Geometry check sheet. Reference: the model listing, model coordinates, mm. A direction names the side the tool comes from. Coordinates: 2 decimals unless noted, no trailing zeros. Loops run counter-clockwise (first coordinate to the right, second up) from the corner with the lowest first, then second, coordinate; pieces in that order, holes last.
from build123d import *

# Parameters (mm, degrees)
EXTRUDE_1_DEPTH            = 1.27
EXTRUDE_2_DEPTH            = 0.01
EXTRUDE_2_DEPTH_BACK       = 10.17
SKETCH_4_R                 = 0.51
SKETCH_4_R_2               = 0.5
CUT_EXTRUDE_1_DEPTH        = 0.1
EXTRUDE_3_DEPTH            = 0.485
PATTERN_LINEAR_1_COUNT     = 3
PATTERN_LINEAR_1_PITCH     = 1.7
PATTERN_LINEAR_1_COL_COUNT = 3
PATTERN_LINEAR_1_COL_PITCH = 1.7


with BuildPart() as part:
    # Эскиз2 → Бобышка-Вытянуть1 (new body)
    with BuildSketch(Plane(origin=(0, 0, 0), x_dir=(1, 0, 0), z_dir=(0, 1, 0))):
        Polygon((3.43, 6.35), (5.08, 6.059060482), (5.08, 5.08), (2.9, 5.08), (2.9, 0), (-2.9, 0), (-2.9, 5.08), (-5.08, 5.08), (-5.08, 6.059060482), (-3.43, 6.35), align=None)
    extrude(amount=EXTRUDE_1_DEPTH)

    # Эскиз3 → Бобышка-Вытянуть2 (add, two sides: drawn at the far end of the back side and taken through both)
    with BuildSketch(Plane.ZY.offset(5.08).offset(-EXTRUDE_2_DEPTH_BACK)):
        Polygon((-5.08, 0.01), (-5.08, 1.27), (-4.673583103, 4.58), (3.357405475, 4.58), (3.56, 2.93), (3.56, 2.55), (3.248127215, 0.01), align=None)
    extrude(amount=EXTRUDE_2_DEPTH + EXTRUDE_2_DEPTH_BACK)

    # Эскиз4 → Вырез-Вытянуть1 (cut)
    with BuildSketch(Plane(origin=(0, 4.58, 0), x_dir=(1, 0, 0), z_dir=(0, 1, 0))):
        with Locations(Location((-3.59, -1.857405475, 0), (0, 0, 270))):
            Circle(SKETCH_4_R)
        with Locations(Location((-3.59, -1.857405475, 0), (0, 0, 270))):
            Circle(SKETCH_4_R_2, mode=Mode.SUBTRACT)
    extrude(amount=-CUT_EXTRUDE_1_DEPTH, mode=Mode.SUBTRACT)

    # Эскиз5 → Бобышка-Вытянуть3 (add, symmetric)
    with BuildSketch(Plane(origin=(0, 0, 0), x_dir=(0, 0, -1), z_dir=(1, 0, 0))):
        with BuildLine():
            Line((-3.56, 2.93), (-3.56, 2.55))
            Line((-3.56, 2.55), (-5.067677126, 2.55))
            ThreePointArc((-5.067677126, 2.55), (-5.576216387, 2.354790067), (-5.823513767, 1.869441632))
            Line((-5.823513767, 1.869441632), (-5.948470433, 0.680558368))
            ThreePointArc((-5.948470433, 0.680558368), (-6.195767813, 0.195209933), (-6.704307074, 0))
            Line((-6.704307074, 0), (-8, 0))
            Line((-8, 0), (-8, 0.38))
            Line((-8, 0.38), (-6.704307074, 0.38))
            ThreePointArc((-6.704307074, 0.38), (-6.450037443, 0.477604966), (-6.326388753, 0.720279184))
            Line((-6.326388753, 0.720279184), (-6.201432087, 1.909162448))
            ThreePointArc((-6.201432087, 1.909162448), (-5.830486018, 2.637185101), (-5.067677126, 2.93))
            Line((-5.067677126, 2.93), (-3.56, 2.93))
        make_face()
    extrude_3 = extrude(amount=EXTRUDE_3_DEPTH, both=True)

    # Линейный массив1: Бобышка-Вытянуть3 ×3
    with Locations(*[(-i * PATTERN_LINEAR_1_PITCH, 0, 0) for i in range(1, PATTERN_LINEAR_1_COUNT)]):
        add(extrude_3)

    # Линейный массив1 col: Бобышка-Вытянуть3 ×3
    with Locations(*[(i * PATTERN_LINEAR_1_COL_PITCH, 0, 0) for i in range(1, PATTERN_LINEAR_1_COL_COUNT)]):
        add(extrude_3)


solid = part.part
(1) Scan lines: L1, parallel to Y at x = 4.75, z = 3; L2, parallel to Y at x = 1.25, z = 3.75; L3, parallel to Z at x = -2, y = 0.75. Record each from-to range of solid material in increasing order.
Findings:
L1: y = 0.01 to 4.58
L2: y = 2.55 to 2.93
L3: z = -6.35 to 3.34, 5.94 to 6.32
(2) Gauge pin test, flat ends, axial feed: pin 1 Ø1.1 at (x, z) = (-3.5, 4.5) entering from +Y; pin 2 Ø1.5 at (y, z) = (1, 5.5) entering from -X (3 decimals); pin 3 Ø0.5 at (x, z) = (-2, 4.5) entering from -Y. Record the tip position at first contact, or that the pin passes through.
Findings:
pin 1: stops at y = 2.93
pin 2: stops at x = -3.885
pin 3: stops at y = 2.55
(3) Access from +Z, -Z, +X, -X, +Y, -Y to the whole of each face (thin tool, end or side, straight path). Record for faces 4 (the flat face through (-3.4, 0.38, 7.4)), 5 (the flat face through (2, 0, 7)), 6 (the flat face through (2, 2.55, 4)), 7 (the flat face through (3.885, 2, 6)), 8 (the flat face through (-3.885, 2, 6)).
Findings:
face 4: +Z, +X, -X, +Y
face 5: +Z, -Z, +X, -X, -Y
face 6: +X, -X, -Y
face 7: +Z, +X, +Y, -Y
face 8: +Z, -X, +Y, -Y
(4) Sectioned sample at A-A on y = 2.1. Record the cut outline in (x, z) (3 decimals).
Findings:
outline: (-5.09, -4.978) - (5.09, -4.978) - (5.09, 3.505) - (-5.09, 3.505) - close; (-3.885, 5.762) - (-2.915, 5.762) - (-2.915, 6.165) - (-3.885, 6.165) - close; (-2.185, 5.762) - (-1.215, 5.762) - (-1.215, 6.165) - (-2.185, 6.165) - close; (-0.485, 5.762) - (0.485, 5.762) - (0.485, 6.165) - (-0.485, 6.165) - close; (1.215, 5.762) - (2.185, 5.762) - (2.185, 6.165) - (1.215, 6.165) - close; (2.915, 5.762) - (3.885, 5.762) - (3.885, 6.165) - (2.915, 6.165) - close
(5) Draft check along X on faces 1 (the flat face through (1.215, 2, 6)), 2 (the flat face through (-5.08, 0.6, -5.6)), 3 (the flat face through (-2, 2.55, 4)). Enter one of: +X half, -X half, draft (parallel to the pull), parting line (faces both ways), or undercut.
Findings:
face 1: undercut
face 2: -X half
face 3: draft
(6) Sectioned sample at C-C on y = 0.95. State how many separate pieces and enclosed holes the cut face has, and give its area (3 significant figures).
Findings:
separate pieces: 6
enclosed holes: 0
area: 100 mm2
